Read the model definition and answer for the solid it produces. Units are mm, in the model's axes. A direction names the side the tool comes from. Give positions to 0.01 mm unless a question says otherwise; leave off trailing zeros. Write each loop counter-clockwise with the first axis right and the second up, starting at its lowest first coordinate (ties: lowest second). Pieces come first, ordered by that corner, then holes. Notation, with made-up numbers: (31.25, 66.25) - (70.25, 66.25) arc R24 ccw to (70.25, 95.25) - close; hole circle Ø6 at (2.25, 73). An arc over 180 degrees is marked (long way). Answer as a JSON object with one key per item and string values. Group by question number.
```python
from build123d import *

# Parameters (mm, degrees)
SKETCH1_R           = 13.75
BOSS_EXTRUDE1_DEPTH = 35.5
SKETCH2_R           = 16.4
BOSS_EXTRUDE2_DEPTH = 3.6
SKETCH3_R           = 10.9
BOSS_EXTRUDE3_DEPTH = 4.4
FILLET1_R           = 3.5
SKETCH4_R           = 0.5
CUT_EXTRUDE1_DEPTH  = 1.3
CHAMFER1_SIZE       = 10
CHAMFER1_SIZE_2     = 1.405408347
FILLET2_R           = 0.5
SKETCH5_W           = 27.8
SKETCH5_H           = 14.4
BOSS_EXTRUDE4_DEPTH = 21
SKETCH6_W           = 10
SKETCH6_H           = 6.3
BOSS_EXTRUDE5_DEPTH = 2.8
SKETCH7_W           = 6.3
SKETCH7_H           = 2.5
CUT_EXTRUDE2_DEPTH  = 9.8
SKETCH8_W           = 6.2
SKETCH8_H           = 0.2
BOSS_EXTRUDE6_DEPTH = 9.6


with BuildPart() as part:
    # Sketch1 → Boss-Extrude1 (new body)
    with BuildSketch(Plane(origin=(0, 0, 0), x_dir=(1, 0, 0), z_dir=(0, 1, 0))):
        with Locations(Location((0, 0, 0), (0, 0, 270))):
            Circle(SKETCH1_R)
    extrude(amount=BOSS_EXTRUDE1_DEPTH)

    # Sketch2 → Boss-Extrude2 (add)
    with BuildSketch(Plane(origin=(0, 35.5, 0), x_dir=(1, 0, 0), z_dir=(0, 1, 0))):
        with Locations(Location((0, 0, 0), (0, 0, 270))):
            Circle(SKETCH2_R)
    extrude(amount=BOSS_EXTRUDE2_DEPTH)

    # Sketch3 → Boss-Extrude3 (add)
    with BuildSketch(Plane(origin=(0, 39.1, 0), x_dir=(1, 0, 0), z_dir=(0, 1, 0))):
        with Locations(Location((0, 0, 0), (0, 0, 270))):
            Circle(SKETCH3_R)
    extrude(amount=BOSS_EXTRUDE3_DEPTH)

    # Fillet1
    fillet1_edges = [part.edges().sort_by_distance(p)[0] for p in [
        (0, 39.1, -16.4),
    ]]
    fillet(fillet1_edges, radius=FILLET1_R)

    # Sketch4 → Cut-Extrude1 (cut)
    with BuildSketch(Plane(origin=(0, 43.5, 0), x_dir=(1, 0, 0), z_dir=(0, 1, 0))):
        with Locations(Location((0, 0, 0), (0, 0, 270))):
            Circle(SKETCH4_R)
    extrude(amount=-CUT_EXTRUDE1_DEPTH, mode=Mode.SUBTRACT)

    # Chamfer1
    # the kernel refuses this chamfer: 10, 1.405408347 mm, written as the material it takes off along each edge
    with BuildSketch(Plane(origin=(0, 43.5, 0), x_dir=(0, 0, 1), z_dir=(-1, 0, 0))) as chamfer1_piece_1_section:
        Polygon((0.5 + CHAMFER1_SIZE, 0), (0.5, -CHAMFER1_SIZE_2), (0.5, 0), align=None)
    chamfer1_piece_1 = revolve(axis=Axis((0, 43.5, 0), (0, 1, 0)), mode=Mode.PRIVATE)
    chamfer1_piece_1 = split(chamfer1_piece_1, bisect_by=Plane(origin=(0, 42.2, -6.064294667), z_dir=(0, 1, 0)), keep=Keep.TOP, mode=Mode.PRIVATE)
    add(chamfer1_piece_1, mode=Mode.SUBTRACT)

    # Fillet2
    # the kernel refuses this fillet: 0.5 mm, written as the material it takes off along each edge
    with BuildSketch(Plane(origin=(0, 43.5, 0), x_dir=(0, 0, 1), z_dir=(-1, 0, 0))) as fillet2_piece_1:
        with BuildLine():
            CenterArc((10.4, -0.489897949), FILLET2_R, 0, 78.463040967)
            Line((10.5, 0), (10.502, 0.009797959))
            ThreePointArc((10.502, 0.009797959), (10.7, 0.01), (10.9, 0.01))
            Line((10.9, 0.01), (10.91, 0))
            Line((10.91, 0), (10.91, -0.489897949))
            Line((10.91, -0.489897949), (10.9, -0.489897949))
        make_face()
    revolve(axis=Axis((0, 43.5, 0), (0, 1, 0)), mode=Mode.SUBTRACT)

    # Sketch5 → Boss-Extrude4 (add)
    with BuildSketch(Plane.XZ):
        Rectangle(SKETCH5_W, SKETCH5_H)
    extrude(amount=BOSS_EXTRUDE4_DEPTH)

    # Sketch6 → Boss-Extrude5 (add)
    with BuildSketch(Plane.XZ.offset(21)):
        with Locations((6.7, 0)):
            Rectangle(SKETCH6_W, SKETCH6_H)
    extrude(amount=BOSS_EXTRUDE5_DEPTH)

    # Sketch7 → Cut-Extrude2 (cut)
    with BuildSketch(Plane(origin=(11.7, 0, 0), x_dir=(0, 0, -1), z_dir=(1, 0, 0))):
        with Locations((0, -22.25)):
            Rectangle(SKETCH7_W, SKETCH7_H)
    extrude(amount=-CUT_EXTRUDE2_DEPTH, mode=Mode.SUBTRACT)

    # Sketch8 → Boss-Extrude6 (add)
    with BuildSketch(Plane(origin=(13.9, 0, 0), x_dir=(0, 0, -1), z_dir=(1, 0, 0))):
        with Locations((0, -17.1)):
            Rectangle(SKETCH8_W, SKETCH8_H)
        with Locations((0, -11.4)):
            Rectangle(SKETCH8_W, SKETCH8_H)
    extrude(amount=BOSS_EXTRUDE6_DEPTH)


solid = part.part
```
1) For a pull along X with two mould halves and no side action, classify faces 6 (the flat face through (0, 42.2, 0)), 7 (the flat face through (1.7, -22, 0)), 8 (the flat face through (19, -17.2, 0)) as released by +X, released by -X, zero draft, split by the parting line, or undercut.
2) Flat-ended cylindrical pins translate along their axes: pin 1 Ø2 at (x, y) = (-4.5, 27) entering from +Z; pin 2 Ø6 at (y, z) = (-3, 1.5) entering from +X; pin 3 Ø1.7 at (x, z) = (-13.5, -1.5) entering from +Y. Find the tip coordinate at first contact, or state that the pin passes through.
3) Find section D-D, the plane y = 28. Write down the section's boundary in (x, z).
4) Find section B-B, the plane x = 0. Write down the section's boundary in (y, z).
5) Find the intervals of material crossed by line 1 (Z direction, x = -3.5, y = -11); line 2 (X direction, y = -8, z = 2.5); line 3 (Y direction, x = -13, z = 0), in increasing order. Write a range as [from, to].
6) Find section A-A, the plane x = 21. Write down the section's boundary in (y, z).
7) Find section C-C, the plane y = -5.5. Write down the section's boundary in (x, z), and give its area (3 significant figures).
8) Which of the six approach directions +Z, -Z, +X, -X, +Y, -Y give full straight-line access (tool end or side, diameter ignored) to faces 1 (the flat face through (-11, 35.5, -9)), 2 (the flat face through (0, -10, 7.2)), 3 (the flat face through (11, 39.1, -3)), 4 (the flat face through (1.9, -22, 0)), 5 (the flat face through (0, -10, -7.2))?
Values follow:
{
 "1": {"face 6": "undercut", "face 7": "released by -X", "face 8": "zero draft"},
 "2": {"pin 1": "stops at z = 13.3", "pin 2": "stops at x = 13.9", "pin 3": "stops at y = 39.1"},
 "3": {"outline": "circle Ø27.5 at (0, 0)"},
 "4": {"outline": "(-21, -7.2) - (0, -7.2) - (0, -13.75) - (35.5, -13.75) - (35.5, -16.4) - (35.6, -16.4) arc R3.5 ccw to (39.1, -12.9) - (39.1, -10.9) - (43.01, -10.9) arc R0.5 ccw to (43.5, -10.5) - (42.2, -1.25) - (42.2, 1.25) - (43.5, 10.5) arc R0.5 ccw to (43.01, 10.9) - (39.1, 10.9) - (39.1, 12.9) arc R3.5 ccw to (35.6, 16.4) - (35.5, 16.4) - (35.5, 13.75) - (0, 13.75) - (0, 7.2) - (-21, 7.2) - close"},
 "5": {"line 1": "z = [-7.2, 7.2]", "line 2": "x = [-13.9, 13.9]", "line 3": "y = [-21, 39.1]"},
 "6": {"outline": "(-17.2, -3.1) - (-17, -3.1) - (-17, 3.1) - (-17.2, 3.1) - close; (-11.5, -3.1) - (-11.3, -3.1) - (-11.3, 3.1) - (-11.5, 3.1) - close"},
 "7": {"outline": "(-13.9, -7.2) - (13.9, -7.2) - (13.9, 7.2) - (-13.9, 7.2) - close", "area": "400 mm2"},
 "8": {"face 1": "none", "face 2": "+Z, +X, -X, -Y", "face 3": "+Y", "face 4": "+Z, -Z, +X", "face 5": "-Z, +X, -X, -Y"}
}
